```python
from build123d import *

# Parameters (mm, degrees)
F0_W     = 1120
F0_H     = 1120
F1_DEPTH = 1040
F2_T     = -5
F3_DEPTH = 160
F4_W     = 1040
F4_H     = 280
F4_H_2   = 160
F5_DEPTH = 1120.001
F6_W     = 1040
F6_H     = 280
F6_H_2   = 160
F7_DEPTH = 1120.001


with BuildPart() as f1:
    # F0 (on Top) → F1 (new body)
    with BuildSketch(Plane.XY):
        Rectangle(F0_W, F0_H)
    extrude(amount=F1_DEPTH)

    # F2
    f2_openings = [f1.faces().sort_by_distance(p)[0] for p in [
        (0, 0, 1040),
    ]]
    offset(amount=F2_T, openings=f2_openings)

    # F0 (on Top) → F3 (join)
    with BuildSketch(Plane.XY):
        Rectangle(F0_W, F0_H)
    extrude(amount=-F3_DEPTH)

    # F4 (on face) → F5 (cut, through all)
    with BuildSketch(Plane.YZ.offset(560)):
        with Locations((0, 900)):
            Rectangle(F4_W, F4_H)
        with Locations((0, -80)):
            Rectangle(F4_W, F4_H_2)
    extrude(amount=-F5_DEPTH, mode=Mode.SUBTRACT)

    # F6 (on face) → F7 (cut, through all)
    with BuildSketch(Plane.XZ.offset(560)):
        with Locations((0, 900)):
            Rectangle(F6_W, F6_H)
        with Locations((0, -80)):
            Rectangle(F6_W, F6_H_2)
    extrude(amount=-F7_DEPTH, mode=Mode.SUBTRACT)


solid = f1.part
```
Could you check a few things on this model? Use its own coordinates, in mm. A direction names the side the tool comes from. Give positions to 0.01 mm unless a question says otherwise; leave off trailing zeros. Loops run counter-clockwise (first coordinate to the right, second up) from the corner with the lowest first, then second, coordinate; pieces in that order, holes last. Notation, with made-up numbers: (1, 80.25) - (45, 80.25) arc R20 cw to (45, 105.25) - close; hole circle Ø9 at (0.5, -19.75). An arc over 180 degrees is marked (long way). Answer in a Markdown table with one row per item. Add a question column.
Q1. If we section it at C-C (z = 140): List the corners of the cut face in (x, y) for me.
Q2. If we section it at A-A (z = 947.5): List the corners of the cut face in (x, y) for me.
Q3. Which directions (+Z, -Z, +X, -X, +Y, -Y) give clear straight access to the entire face, cutting with the end or side of a thin tool? Please do faces 5 (the face through (549, -556, 1040)), 6 (the face through (555, -8, 400)), 7 (the face through (540, 520, -81)), 8 (the face through (-520, -540, -81)).
Q4. For pin 1 (4 mm diameter, centred on x = -216.5, y = -558.5, fed in from +Z); pin 2 (1 mm diameter, centred on x = -354.5, y = 45, fed in from +Z), each with a flat end and sliding along its axis, tell me the tip position at first contact or that it passes through.
Q5. Please list where these lines run through material, in increasing order: L1, parallel to Y at x = -365, z = 265; L2, parallel to Z at x = 172.5, y = 358. Write a range as from..to.
Q6. If we section it at B-B (x = -197.5): List the corners of the cut face in (y, z) for me, plus the area to 4 significant figures.
Q7. We'd pull the mould along X, two halves only. Please class faces 1 (the face through (-560, -8, 448)), 2 (the face through (540, 540, -160)), 3 (the face through (-8, 555, 400)), 4 (the face through (520, -540, -81)): +X half, -X half, draft (parallel to the pull), parting line (faces both ways), or undercut.
The answers:
| question | item | result |
|---|---|---|
| 1 | outline | (-560, -560) - (560, -560) - (560, 560) - (-560, 560) - close; hole (-555, -555) - (555, -555) - (555, 555) - (-555, 555) - close |
| 2 | outline | (-560, -560) - (-520, -560) - (-520, -555) - (-555, -555) - (-555, -520) - (-560, -520) - close; (-560, 520) - (-555, 520) - (-555, 555) - (-520, 555) - (-520, 560) - (-560, 560) - close; (520, -560) - (560, -560) - (560, -520) - (555, -520) - (555, -555) - (520, -555) - close; (520, 555) - (555, 555) - (555, 520) - (560, 520) - (560, 560) - (520, 560) - close |
| 3 | face 5 | +Z, +X, -X, +Y, -Y |
| 3 | face 6 | +Z |
| 3 | face 7 | -Z, +X, -X |
| 3 | face 8 | -Z, +Y, -Y |
| 4 | pin 1 | stops at z = 760 |
| 4 | pin 2 | stops at z = 5 |
| 5 | L1 | y = -560..-555, 555..560 |
| 5 | L2 | z = 0..5 |
| 6 | outline | (-560, 0) - (560, 0) - (560, 760) - (555, 760) - (555, 5) - (-555, 5) - (-555, 760) - (-560, 760) - close |
| 6 | area | 13,150 mm^2 |
| 7 | face 1 | -X half |
| 7 | face 2 | draft |
| 7 | face 3 | undercut |
| 7 | face 4 | undercut |
